For this review, use the dimensioned drawing (mm, ordinates from the lowest corner) and the shaded views. A direction names the side the tool comes from. Give positions to 0.01 mm unless a question says otherwise; leave off trailing zeros. Write each loop counter-clockwise with the first axis right and the second up, starting at its lowest first coordinate (ties: lowest second). Pieces come first, ordered by that corner, then holes. Notation, with made-up numbers: M -4,52.25 L 26,52.25 A32 ccw 26,88.25 Z; hole C 80.25,43 d5. An arc over 180 degrees is marked long. One line per item, written item: value. Start each with the question number.
Item 1: Consider section B-B, the plane z = 9.25. Write out the cut boundary in (x, y).
Item 2: Tool access review of the marked faces 5, 6 and 7: name each direction out of +Z, -Z, +X, -X, +Y, -Y from which nothing blocks a thin tool from reaching the whole face with its end or side.
Item 3: Mouldability with a two-part tool opening along Z and no side actions: class the marked faces 1, 2, 3 and 4 as released by +Z, released by -Z, zero draft, split by the parting line, or undercut.
Item 4: Clearance check with flat-ended pins moving along their axes: pin 1 Ø1 at (x, z) = (10, 13) entering from +Y; pin 2 Ø1.5 at (y, z) = (13.5, 10) entering from -X; pin 3 Ø0.6 at (x, z) = (11.5, 13.5) entering from -Y; pin 4 Ø6 at (x, z) = (16, 5.5) entering from -Y. State where each tip first meets the part, or that it passes through.
Item 5: Consider section C-C, the plane z = 6.5. Write out the cut boundary in (x, y), and give its area (3 significant figures).
Item 6: To check wall thickness, follow probe 1 along Z at (x, y) = (4, 10.25); probe 2 along Y at (x, z) = (17, 4.75); probe 3 along Y at (x, z) = (2.5, 4.5). State the ranges of each line that lie inside material, in increasing order.
Item 7: Consider section A-A, the plane y = 9.5. Write out the cut boundary in (x, z).
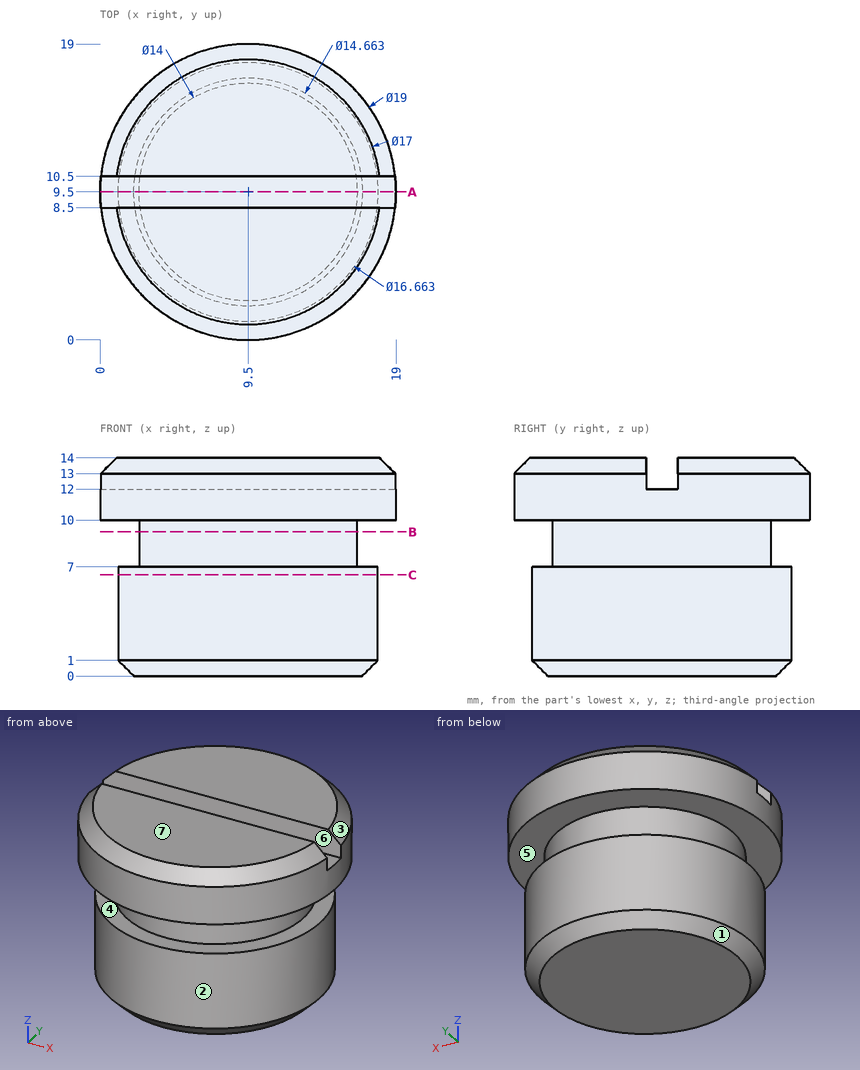
Model answer:
1. outline: C 9.5,9.5 d14
2. face 5: none
2. face 6: +Z, +X, -X
2. face 7: +Z, +X, -X, +Y, -Y
3. face 1: released by -Z
3. face 2: zero draft
3. face 3: released by +Z
3. face 4: undercut
4. pin 1: stops at y = 19
4. pin 2: stops at x = 0.57
4. pin 3: stops at y = 0.41
4. pin 4: stops at y = 1.94
5. outline: C 9.5,9.5 d16.66
5. area: 218 mm2
6. probe 1: z = 0 to 12
6. probe 2: y = 5.87 to 13.13
6. probe 3: y = 4.98 to 14.02
7. outline: M 0,10 L 2.5,10 L 2.5,7 L 1.17,7 L 1.17,1 L 2.17,0 L 16.83,0 L 17.83,1 L 17.83,7 L 16.5,7 L 16.5,10 L 19,10 L 19,12 L 0,12 Z
